Design review of the part built by this model. Coordinates are the model's own, in mm. A direction names the side the tool comes from. Coordinates: 2 decimals unless noted, no trailing zeros. Loops run counter-clockwise (first coordinate to the right, second up) from the corner with the lowest first, then second, coordinate; pieces in that order, holes last. Notation, with made-up numbers: (-19.5, 42.25) -> (27.5, 42.25) arc R25 cw to (27.5, 77.25) -> close; hole circle Ø11 at (43.25, 81.25). An arc over 180 degrees is marked (long way). Answer in a Markdown table with one row per item.
```python
from build123d import *

# Parameters (mm, degrees)
SKETCH_W     = 60
SKETCH_H     = 25
SKETCH_R     = 3.3
PAD_DEPTH    = 36
SKETCH001_W  = 60
SKETCH001_H  = 22.1
PAD001_DEPTH = 127
SKETCH002_R  = 2.5
POCKET_DEPTH = 22.101
PAD002_DEPTH = 60
SKETCH004_W  = 152
SKETCH004_H  = 32.1
PAD003_DEPTH = 10
SKETCH005_W  = 152
SKETCH005_H  = 32.1
PAD004_DEPTH = 10
PAD005_DEPTH = 25
SKETCH007_W  = 60
SKETCH007_H  = 15
PAD006_DEPTH = 12
PAD007_DEPTH = 60


with BuildPart() as part:
    # Sketch → Pad (new body)
    with BuildSketch(Plane.XY):
        Rectangle(SKETCH_W, SKETCH_H)
        with Locations((-23, 6.5)):
            Circle(SKETCH_R, mode=Mode.SUBTRACT)
        with Locations((-23, -6.5)):
            Circle(SKETCH_R, mode=Mode.SUBTRACT)
        with Locations((23, -6.5)):
            Circle(SKETCH_R, mode=Mode.SUBTRACT)
        with Locations((23, 6.5)):
            Circle(SKETCH_R, mode=Mode.SUBTRACT)
    extrude(amount=PAD_DEPTH)

    # Sketch001 (on Face1 of Pad) → Pad001 (join)
    with BuildSketch(Plane(origin=(0, 12.5, 0), x_dir=(-1, 0, 0), z_dir=(0, 1, 0))):
        with Locations((0, 11.05)):
            Rectangle(SKETCH001_W, SKETCH001_H)
    extrude(amount=PAD001_DEPTH)

    # Sketch002 (on Face2 of Pad001) → Pocket (cut, through all)
    with BuildSketch(Plane.XY.offset(22.1)):
        with Locations((-20, 124.5)):
            Circle(SKETCH002_R)
        with Locations((20, 124.5)):
            Circle(SKETCH002_R)
        with Locations((-20, 90.5)):
            Circle(SKETCH002_R)
        with Locations((20, 90.5)):
            Circle(SKETCH002_R)
    extrude(amount=-POCKET_DEPTH, mode=Mode.SUBTRACT)

    # Sketch003 (on Face6 of Pocket) → Pad002 (join)
    with BuildSketch(Plane.YZ.offset(30)):
        Polygon((12.5, 36), (32.5, 22.1), (12.5, 0), align=None)
    extrude(amount=-PAD002_DEPTH)

    # Sketch004 (on Face7 of Pad002) → Pad003 (join)
    with BuildSketch(Plane.YZ.offset(30)):
        with Locations((63.5, 6.05)):
            Rectangle(SKETCH004_W, SKETCH004_H)
    extrude(amount=PAD003_DEPTH)

    # Sketch005 (on Face20 of Pad003) → Pad004 (join)
    with BuildSketch(Plane(origin=(-30, 0, 0), x_dir=(0, -1, 0), z_dir=(-1, 0, 0))):
        with Locations((-63.5, 6.05)):
            Rectangle(SKETCH005_W, SKETCH005_H)
    extrude(amount=PAD004_DEPTH)

    # Sketch006 (on Face3 of Pad004) → Pad005 (join)
    with BuildSketch(Plane.XZ.offset(12.5)):
        Polygon((40, 22.1), (30, 22.1), (30, 36), align=None)
        Polygon((-30, 36), (-30, 22.1), (-40, 22.1), align=None)
    extrude(amount=-PAD005_DEPTH)

    # Sketch007 (on Face25 of Pad005) → Pad006 (join)
    with BuildSketch(Plane.XZ.offset(12.5)):
        with Locations((0, 7.5)):
            Rectangle(SKETCH007_W, SKETCH007_H)
    extrude(amount=PAD006_DEPTH)

    # Sketch008 (on Face40 of Pad006) → Pad007 (join)
    with BuildSketch(Plane(origin=(-30, 0, 0), x_dir=(0, -1, 0), z_dir=(-1, 0, 0))):
        Polygon((24.5, 15), (12.5, 15), (12.5, 22.1), align=None)
    extrude(amount=-PAD007_DEPTH)


solid = part.part
```
(1) Take a section at C-C on x = 14. Give the boundary of the cut face in (y, z), and give its area (3 significant figures).
Evaluation:
| item | result |
|---|---|
| outline | (-24.5, 0) -> (139.5, 0) -> (139.5, 22.1) -> (32.5, 22.1) -> (12.5, 36) -> (-12.5, 36) -> (-12.5, 22.1) -> (-24.5, 15) -> close |
| area | 4,070 mm² |
(2) Take a section at D-D on z = 3. Count the separate pieces of the cut face and the enclosed holes in it, and give its area (3 significant figures).
Evaluation:
| item | result |
|---|---|
| separate pieces | 1 |
| enclosed holes | 8 |
| area | 12,700 mm² |
(3) Tool access review of faces 5 (the flat face through (30, -19, 9)), 6 (the flat face through (30, 62, -5)), 7 (the flat face through (-30, 18, 26)): name each direction out of +Z, -Z, +X, -X, +Y, -Y from which nothing blocks a thin tool from reaching the whole face with its end or side.
Evaluation:
| item | result |
|---|---|
| face 5 | +Z, -Z, +X, -Y |
| face 6 | -Z, +Y, -Y |
| face 7 | +Z, -X, +Y |
(4) Draft analysis for pull direction X (two halves, no side actions). For faces 1 (the flat face through (0, 59, 0)), 2 (the flat face through (1, -12.5, 24)), 3 (the flat face through (30, 18, 26)), 4 (the cylindrical face through (-19.85, 7.49, 17.75)), state which applies: pulls with the +X half, pulls with the -X half, needs draft (parallel to the pull), parting line crosses it, or undercut.
Evaluation:
| item | result |
|---|---|
| face 1 | undercut |
| face 2 | needs draft |
| face 3 | pulls with the +X half |
| face 4 | undercut |
(5) For pin 1 (10.5 mm diameter, centred on x = -23, y = 6.5, fed in from +Z); pin 2 (8 mm diameter, centred on x = 8, y = 71, fed in from +Z); pin 3 (10.5 mm diameter, centred on x = 23, y = 6.5, fed in from -Z); pin 4 (6 mm diameter, centred on x = 24.5, y = 30.5, fed in from +Z) (3 decimals), all flat-tipped, find the tip position at first contact; note any pin that passes through.
Evaluation:
| item | result |
|---|---|
| pin 1 | stops at z = 36 |
| pin 2 | stops at z = 22.1 |
| pin 3 | stops at z = 0 |
| pin 4 | stops at z = 25.575 |
(6) Take a section at B-B on y = 90.5. Give the boundary of the cut face in (x, z).
Evaluation:
| item | result |
|---|---|
| outline | (-40, -10) -> (-30, -10) -> (-30, 0) -> (-22.5, 0) -> (-22.5, 22.1) -> (-40, 22.1) -> close; (-17.5, 0) -> (17.5, 0) -> (17.5, 22.1) -> (-17.5, 22.1) -> close; (22.5, 0) -> (30, 0) -> (30, -10) -> (40, -10) -> (40, 22.1) -> (22.5, 22.1) -> close |
(7) Take a section at A-A on z = -5. Give the boundary of the cut face in (x, y), and give its area (3 significant figures).
Evaluation:
| item | result |
|---|---|
| outline | (-40, -12.5) -> (-30, -12.5) -> (-30, 139.5) -> (-40, 139.5) -> close; (30, -12.5) -> (40, -12.5) -> (40, 139.5) -> (30, 139.5) -> close |
| area | 3,040 mm² |
(8) To check wall thickness, follow probe 1 along X at (y, z) = (-6, 15); probe 2 along X at (y, z) = (92, 7); probe 3 along Y at (x, z) = (20, 17.25). State the ranges of each line that lie inside material, in increasing order.
Evaluation:
| item | result |
|---|---|
| probe 1 | x = -40 to -26.26, -19.74 to 19.74, 26.26 to 40 |
| probe 2 | x = -40 to -22, -18 to 18, 22 to 40 |
| probe 3 | y = -20.7 to -7.87, -5.13 to 5.13, 7.87 to 88, 93 to 122, 127 to 139.5 |
